Print and shaded views of the part. All mm, measured from the part's lowest x, y and z. A direction names the side the tool comes from. Give positions to 0.01 mm unless a question says otherwise; leave off trailing zeros. Loops run counter-clockwise (first coordinate to the right, second up) from the corner with the lowest first, then second, coordinate; pieces in that order, holes last. Notation, with made-up numbers: (23, 36) -> (32, 36) arc R33 ccw to (32, 68) -> close; hole circle Ø3 at (78.25, 16). An arc over 180 degrees is marked (long way). Write each question's results on one line, items separated by ' | '. Start each with the question number.
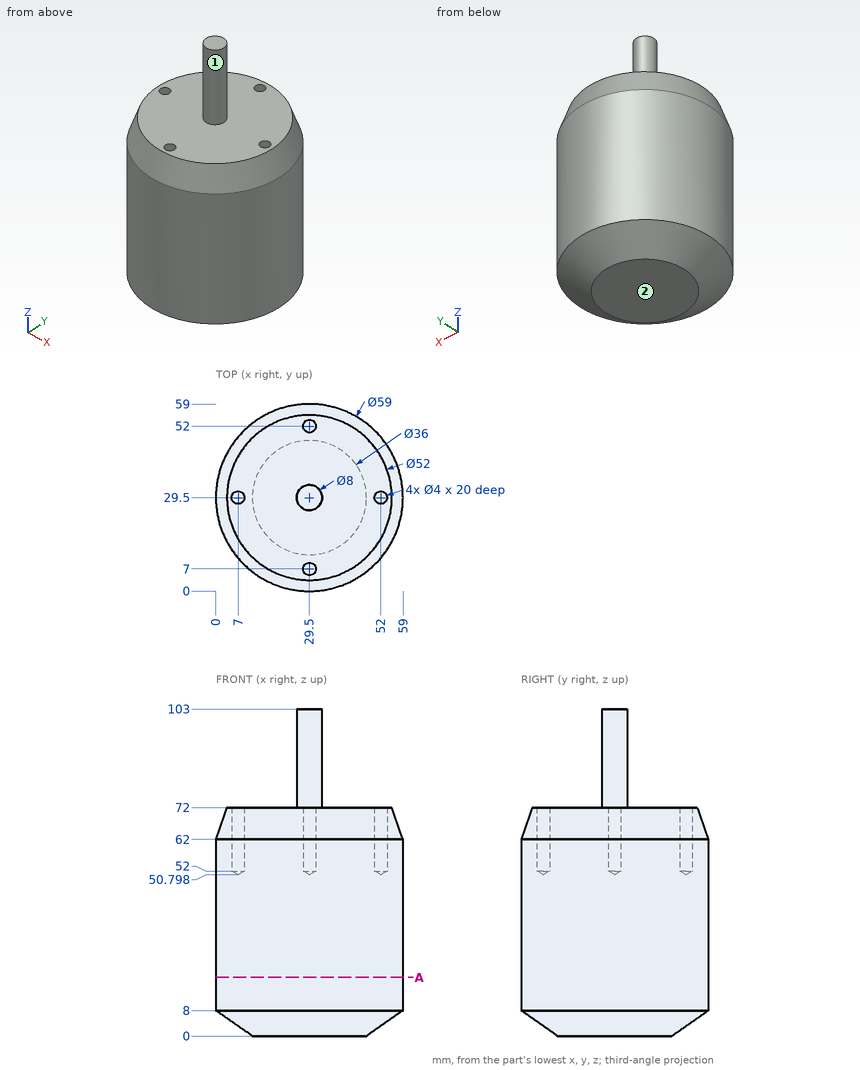
Q1. Saw through at A-A, the plane z = 18.5. List the corners of the cut face in (x, y), then the cut area to 3 significant figures.
Q2. Which spindle directions (+Z, -Z, +X, -X, +Y, -Y) get a long thin tool onto all of the face, cutting with end or side? Do the marked faces 1 and 2. Say none if no direction does.
Q3. Wall check: L1, parallel to X at y = 29.5, z = 68; L2, parallel to Z at x = 34, y = 43; L3, parallel to X at y = 7, z = 63.5 (1 decimal). Give the ranges that are in metal, low to high.
Q4. Drop flat-ended pins along their axis: pin 1 (6 mm diameter, centred on x = 40.5, y = 30.5, fed in from +Z); pin 2 (8 mm diameter, centred on y = 10, z = 11.5, fed in from +X); pin 3 (15.5 mm diameter, centred on x = 29.5, y = 23.5, fed in from +Z); pin 4 (12 mm diameter, centred on x = 43.5, z = 84.5, fed in from -Y). Give the stop position or say it passes through.
Answer block:
1) outline: circle Ø59 at (29.5, 29.5) | area: 2,730 mm2
2) face 1: +Z | face 2: -Z, +X, -X, +Y, -Y
3) L1: x = 2.1 to 5, 9 to 50, 54 to 56.9 | L2: z = 0 to 72 | L3: x = 11.2 to 27.5, 31.5 to 47.8
4) pin 1: stops at z = 72 | pin 2: stops at x = 54.6 | pin 3: stops at z = 103 | pin 4: passes through
